Design review of the part shown in the three views and the two pictorial views. Dimensions are in mm from the part's minimum x, y and z. A direction names the side the tool comes from. Coordinates: 2 decimals unless noted, no trailing zeros. Loops run counter-clockwise (first coordinate to the right, second up) from the corner with the lowest first, then second, coordinate; pieces in that order, holes last. Notation, with made-up numbers: (7.25, -13.75) -> (11.25, -13.75) arc R23 ccw to (11.25, 11.25) -> close; hole circle Ø5 at (60.25, -14.5). An arc over 180 degrees is marked (long way). One line per item, written item: value.
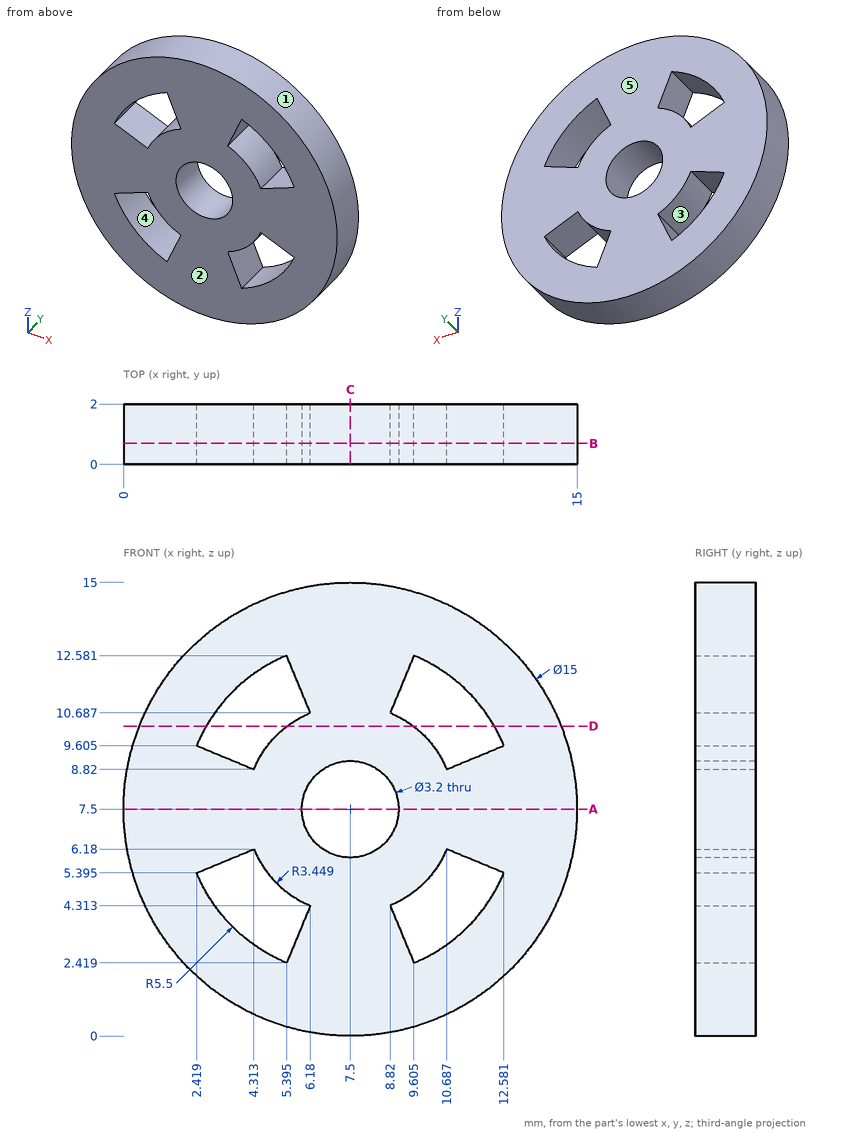
1. For the marked faces 4 and 5, list the 3-axis set-ups (+Z, -Z, +X, -X, +Y, -Y) from which the entire face can be reached by the end or side of a thin tool; tool diameter is ignored.
Return value:
face 4: +Y, -Y
face 5: +Z, -Z, +X, -X, +Y
2. Take a section at D-D, the plane z = 10.25. Give the boundary of the cut face in (x, y).
Return value:
outline: (0.52, 0) -> (2.74, 0) -> (2.74, 2) -> (0.52, 2) -> close; (5.42, 0) -> (9.58, 0) -> (9.58, 2) -> (5.42, 2) -> close; (12.26, 0) -> (14.48, 0) -> (14.48, 2) -> (12.26, 2) -> close
3. To check wall thickness, follow probe 1 along X at (y, z) = (0.7, 7.5); probe 2 along X at (y, z) = (0.85, 3.75) (1 decimal); probe 3 along X at (y, z) = (0.1, 10.5) (1 decimal). State the ranges of each line that lie inside material, in increasing order. Write a range as from..to.
Return value:
probe 1: x = 0..5.9, 9.1..15
probe 2: x = 1..3.5, 5.9..9.1, 11.5..14
probe 3: x = 0.6..2.9, 5.8..9.2, 12.1..14.4
4. Insertion check: pin 1 Ø1 at (y, z) = (0.5, 11.5) entering from +X. The pin has a flat end and moves straight along its axis. Give the tip position at first contact, or say it passes through.
Return value:
pin 1: stops at x = 14.13
5. Take a section at A-A, the plane z = 7.5. Give the boundary of the cut face in (x, y).
Return value:
outline: (0, 0) -> (5.9, 0) -> (5.9, 2) -> (0, 2) -> close; (9.1, 0) -> (15, 0) -> (15, 2) -> (9.1, 2) -> close
6. The part is to be moulded in two halves that separate along Z. For the marked faces 1, 2 and 3, say which applies: pulls with the +Z half, pulls with the -Z half, needs draft (parallel to the pull), parting line crosses it, or undercut.
Return value:
face 1: parting line crosses it
face 2: needs draft
face 3: undercut
7. Take a section at B-B, the plane y = 0.7. Give the number of separate pieces and of enclosed holes in the cut face, and give its area (3 significant figures).
Return value:
separate pieces: 1
enclosed holes: 5
area: 140 mm2
8. Take a section at C-C, the plane x = 7.5. Give the boundary of the cut face in (y, z), and give its area (3 significant figures).
Return value:
outline: (0, 0) -> (2, 0) -> (2, 5.9) -> (0, 5.9) -> close; (0, 9.1) -> (2, 9.1) -> (2, 15) -> (0, 15) -> close
area: 23.6 mm2
